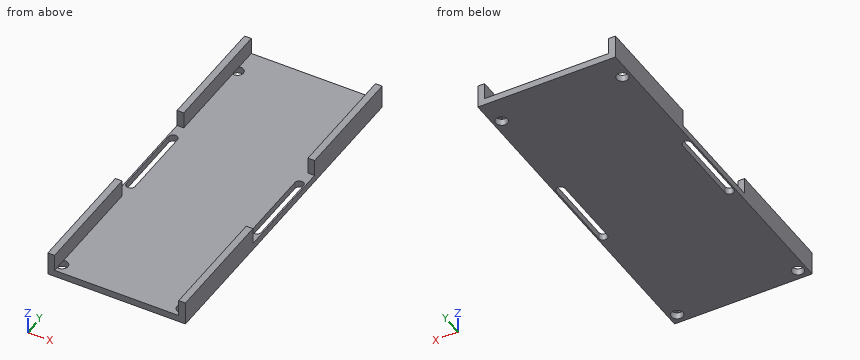
```python
from build123d import *

# Parameters (mm, degrees)
FLOOR_AND_STRAP_GUIDES_PROFILE_W = 41
FLOOR_AND_STRAP_GUIDES_PROFILE_H = 102
FLOOR_AND_STRAP_GUIDES_PROFILE_R = 1.75
FLOOR_AND_STRAP_GUIDES_DEPTH     = 2
INTEGRAL_START                   = 2
INTEGRAL_EDGE_STOPS_PROFILE_W    = 2
INTEGRAL_EDGE_STOPS_PROFILE_H    = 35
INTEGRAL_EDGE_STOPS_DEPTH        = 5


with BuildPart() as part:
    # Floor and strap guides profile → Floor and strap guides (new body)
    with BuildSketch(Plane.XY):
        Rectangle(FLOOR_AND_STRAP_GUIDES_PROFILE_W, FLOOR_AND_STRAP_GUIDES_PROFILE_H)
        with Locations((-18, -48)):
            Circle(FLOOR_AND_STRAP_GUIDES_PROFILE_R, mode=Mode.SUBTRACT)
        with Locations((-18, 43)):
            Circle(FLOOR_AND_STRAP_GUIDES_PROFILE_R, mode=Mode.SUBTRACT)
        with Locations((18, -48)):
            Circle(FLOOR_AND_STRAP_GUIDES_PROFILE_R, mode=Mode.SUBTRACT)
        with Locations((18, 43)):
            Circle(FLOOR_AND_STRAP_GUIDES_PROFILE_R, mode=Mode.SUBTRACT)
        with BuildLine():
            Line((-17.5, -11), (-17.5, 11))
            ThreePointArc((-17.5, 11), (-18.8, 12.3), (-20.1, 11))
            Line((-20.1, 11), (-20.1, -11))
            ThreePointArc((-20.1, -11), (-18.8, -12.3), (-17.5, -11))
        make_face(mode=Mode.SUBTRACT)
        with BuildLine():
            Line((20.1, -11), (20.1, 11))
            ThreePointArc((20.1, 11), (18.8, 12.3), (17.5, 11))
            Line((17.5, 11), (17.5, -11))
            ThreePointArc((17.5, -11), (18.8, -12.3), (20.1, -11))
        make_face(mode=Mode.SUBTRACT)
    extrude(amount=FLOOR_AND_STRAP_GUIDES_DEPTH)

    # Integral edge stops profile → Integral edge stops (add)
    with BuildSketch(Plane.XY.offset(INTEGRAL_START)):
        with Locations((-19.5, -33.5)):
            Rectangle(INTEGRAL_EDGE_STOPS_PROFILE_W, INTEGRAL_EDGE_STOPS_PROFILE_H)
        with Locations((19.5, -33.5)):
            Rectangle(INTEGRAL_EDGE_STOPS_PROFILE_W, INTEGRAL_EDGE_STOPS_PROFILE_H)
        with Locations((-19.5, 33.5)):
            Rectangle(INTEGRAL_EDGE_STOPS_PROFILE_W, INTEGRAL_EDGE_STOPS_PROFILE_H)
        with Locations((19.5, 33.5)):
            Rectangle(INTEGRAL_EDGE_STOPS_PROFILE_W, INTEGRAL_EDGE_STOPS_PROFILE_H)
    extrude(amount=INTEGRAL_EDGE_STOPS_DEPTH)


solid = part.part
```
Can you work these out from the model? Positions are in its coordinate system, mm. Coordinates: 2 decimals unless noted, no trailing zeros. Order: outer loops, then holes, each group sorted by start corner. A loop starts at its lowest first (then second) coordinate and runs counter-clockwise, first axis right, second up.
1. If we section it at C-C (x = 8): Please give me the cut outline in (y, z), then the cut area to 3 significant figures.
2. If we section it at A-A (y = -48): Please give me the cut outline in (x, z).
3. I'm going to push flat-ended pins straight in: pin 1 (0.6 mm diameter, centred on x = -19, y = 42.5, fed in from -Z); pin 2 (10 mm diameter, centred on x = -15, y = 1.5, fed in from +Z). Where does each tip first touch, or does it pass through?
4. If we section it at B-B (z = 3.5): Please give me the cut outline in (x, y), then the cut area to 3 significant figures.
5. I need wall thicknesses on line 1 (X direction, y = 10.5, z = 1); line 2 (X direction, y = 22, z = 4.5); line 3 (Y direction, x = 18, z = 0.5). Which ranges of each line are inside material? Lowest first, please.
Entries:
1. outline: (-51, 0) - (51, 0) - (51, 2) - (-51, 2) - close
1. area: 204 mm2
2. outline: (-20.5, 0) - (-19.75, 0) - (-19.75, 2) - (-18.5, 2) - (-18.5, 7) - (-20.5, 7) - close; (-16.25, 0) - (16.25, 0) - (16.25, 2) - (-16.25, 2) - close; (18.5, 2) - (19.75, 2) - (19.75, 0) - (20.5, 0) - (20.5, 7) - (18.5, 7) - close
3. pin 1: stops at z = 2
3. pin 2: stops at z = 2
4. outline: (-20.5, -51) - (-18.5, -51) - (-18.5, -16) - (-20.5, -16) - close; (-20.5, 16) - (-18.5, 16) - (-18.5, 51) - (-20.5, 51) - close; (18.5, -51) - (20.5, -51) - (20.5, -16) - (18.5, -16) - close; (18.5, 16) - (20.5, 16) - (20.5, 51) - (18.5, 51) - close
4. area: 280 mm2
5. line 1: x = -20.5 to -20.1, -17.5 to 17.5, 20.1 to 20.5
5. line 2: x = -20.5 to -18.5, 18.5 to 20.5
5. line 3: y = -51 to -49.75, -46.25 to -12.02, 12.02 to 41.25, 44.75 to 51
